The listing builds one solid part. Answer for the finished solid, in the listing's coordinates (mm). Round coordinates to 2 decimals unless told otherwise and drop trailing zeros. Order: outer loops, then holes, each group sorted by start corner. A loop starts at its lowest first (then second) coordinate and runs counter-clockwise, first axis right, second up. Notation, with made-up numbers: (21.5, -0.75) - (27.5, -0.75) arc R19 cw to (27.5, 7.25) - close; hole circle Ø8 at (57.25, -31.75). An arc over 180 degrees is marked (long way). Write item = value, one per line.
from build123d import *

# Parameters (mm, degrees)
SKETCH_W  = 200
SKETCH_H  = 80
SKETCH_R  = 2.5
PAD_DEPTH = 1.8


with BuildPart() as part:
    # Sketch → Pad (new body)
    with BuildSketch(Plane.XY):
        with Locations((90, 34.5)):
            Rectangle(SKETCH_W, SKETCH_H)
        Circle(SKETCH_R, mode=Mode.SUBTRACT)
        with Locations((0, 20)):
            Circle(SKETCH_R, mode=Mode.SUBTRACT)
        with Locations((0, 40)):
            Circle(SKETCH_R, mode=Mode.SUBTRACT)
        with Locations((0, 60)):
            Circle(SKETCH_R, mode=Mode.SUBTRACT)
        with Locations((20, 10)):
            Circle(SKETCH_R, mode=Mode.SUBTRACT)
        with Locations((20, 30)):
            Circle(SKETCH_R, mode=Mode.SUBTRACT)
        with Locations((20, 50)):
            Circle(SKETCH_R, mode=Mode.SUBTRACT)
        with Locations((20, 70)):
            Circle(SKETCH_R, mode=Mode.SUBTRACT)
        with Locations((40, 0)):
            Circle(SKETCH_R, mode=Mode.SUBTRACT)
        with Locations((40, 20)):
            Circle(SKETCH_R, mode=Mode.SUBTRACT)
        with Locations((40, 40)):
            Circle(SKETCH_R, mode=Mode.SUBTRACT)
        with Locations((40, 60)):
            Circle(SKETCH_R, mode=Mode.SUBTRACT)
        with Locations((60, 10)):
            Circle(SKETCH_R, mode=Mode.SUBTRACT)
        with Locations((60, 30)):
            Circle(SKETCH_R, mode=Mode.SUBTRACT)
        with Locations((60, 50)):
            Circle(SKETCH_R, mode=Mode.SUBTRACT)
        with Locations((60, 70)):
            Circle(SKETCH_R, mode=Mode.SUBTRACT)
        with Locations((80, 0)):
            Circle(SKETCH_R, mode=Mode.SUBTRACT)
        with Locations((80, 20)):
            Circle(SKETCH_R, mode=Mode.SUBTRACT)
        with Locations((80, 40)):
            Circle(SKETCH_R, mode=Mode.SUBTRACT)
        with Locations((80, 60)):
            Circle(SKETCH_R, mode=Mode.SUBTRACT)
        with Locations((100, 10)):
            Circle(SKETCH_R, mode=Mode.SUBTRACT)
        with Locations((100, 30)):
            Circle(SKETCH_R, mode=Mode.SUBTRACT)
        with Locations((100, 50)):
            Circle(SKETCH_R, mode=Mode.SUBTRACT)
        with Locations((100, 70)):
            Circle(SKETCH_R, mode=Mode.SUBTRACT)
        with Locations((120, 0)):
            Circle(SKETCH_R, mode=Mode.SUBTRACT)
        with Locations((120, 20)):
            Circle(SKETCH_R, mode=Mode.SUBTRACT)
        with Locations((120, 40)):
            Circle(SKETCH_R, mode=Mode.SUBTRACT)
        with Locations((120, 60)):
            Circle(SKETCH_R, mode=Mode.SUBTRACT)
        with Locations((140, 10)):
            Circle(SKETCH_R, mode=Mode.SUBTRACT)
        with Locations((140, 30)):
            Circle(SKETCH_R, mode=Mode.SUBTRACT)
        with Locations((140, 50)):
            Circle(SKETCH_R, mode=Mode.SUBTRACT)
        with Locations((140, 70)):
            Circle(SKETCH_R, mode=Mode.SUBTRACT)
        with Locations((160, 0)):
            Circle(SKETCH_R, mode=Mode.SUBTRACT)
        with Locations((160, 20)):
            Circle(SKETCH_R, mode=Mode.SUBTRACT)
        with Locations((160, 40)):
            Circle(SKETCH_R, mode=Mode.SUBTRACT)
        with Locations((160, 60)):
            Circle(SKETCH_R, mode=Mode.SUBTRACT)
        with Locations((180, 10)):
            Circle(SKETCH_R, mode=Mode.SUBTRACT)
        with Locations((180, 30)):
            Circle(SKETCH_R, mode=Mode.SUBTRACT)
        with Locations((180, 50)):
            Circle(SKETCH_R, mode=Mode.SUBTRACT)
        with Locations((180, 70)):
            Circle(SKETCH_R, mode=Mode.SUBTRACT)
    extrude(amount=PAD_DEPTH)


solid = part.part
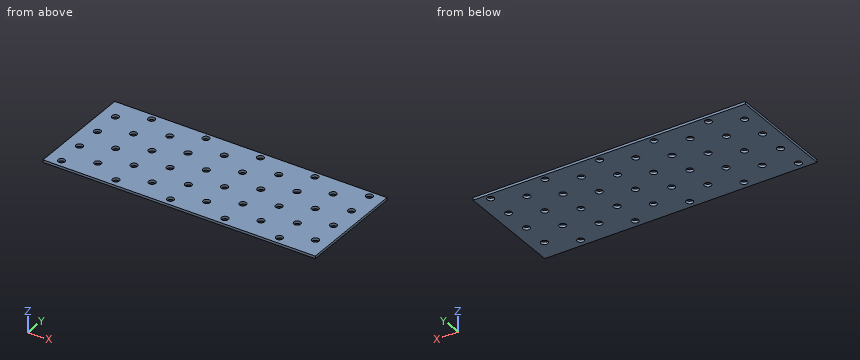
Q1. Section A-A on y = 40 is taken. Determine the outline of the cut face in (x, z), then the cut area to 3 significant figures.
Model answer:
outline = (-10, 0) - (-2.5, 0) - (-2.5, 1.8) - (-10, 1.8) - close; (2.5, 0) - (37.5, 0) - (37.5, 1.8) - (2.5, 1.8) - close; (42.5, 0) - (77.5, 0) - (77.5, 1.8) - (42.5, 1.8) - close; (82.5, 0) - (117.5, 0) - (117.5, 1.8) - (82.5, 1.8) - close; (122.5, 0) - (157.5, 0) - (157.5, 1.8) - (122.5, 1.8) - close; (162.5, 0) - (190, 0) - (190, 1.8) - (162.5, 1.8) - close
area = 315 mm^2
Q2. Section B-B on x = 20 is taken. Determine the outline of the cut face in (y, z).
Model answer:
outline = (-5.5, 0) - (7.5, 0) - (7.5, 1.8) - (-5.5, 1.8) - close; (12.5, 0) - (27.5, 0) - (27.5, 1.8) - (12.5, 1.8) - close; (32.5, 0) - (47.5, 0) - (47.5, 1.8) - (32.5, 1.8) - close; (52.5, 0) - (67.5, 0) - (67.5, 1.8) - (52.5, 1.8) - close; (72.5, 0) - (74.5, 0) - (74.5, 1.8) - (72.5, 1.8) - close
Q3. Section C-C on z = 1.25 is taken. Count the separate pieces of the cut face and the enclosed holes in it, then the cut area to 3 significant figures.
Model answer:
separate_pieces = 1
enclosed_holes = 40
area = 15,200 mm^2
Q4. Find the intervals of material crossed by line 1 (Y direction, x = 160, z = 0.7); line 2 (Y direction, x = 100, z = 0.65); line 3 (X direction, y = 30.5, z = 0.3), in increasing order. Write a range as from..to.
Model answer:
line_1 = -5.5..-2.5, 2.5..17.5, 22.5..37.5, 42.5..57.5, 62.5..74.5
line_2 = -5.5..7.5, 12.5..27.5, 32.5..47.5, 52.5..67.5, 72.5..74.5
line_3 = -10..17.55, 22.45..57.55, 62.45..97.55, 102.45..137.55, 142.45..177.55, 182.45..190
Q5. A flat-ended cylindrical pin translates along its axis: P1, Ø4, axis at x = 100, y = 30, coming from the -Z side. Find the tip coordinate at first contact, or state that the pin passes through.
Model answer:
P1 = through
